Geometry: final body of the model. Coordinates: model frame, mm. A direction names the side the tool comes from. Give positions to 0.01 mm unless a question says otherwise; leave off trailing zeros. Order: outer loops, then holes, each group sorted by start corner. A loop starts at its lowest first (then second) coordinate and runs counter-clockwise, first axis right, second up. Notation, with made-up numbers: (0.25, -24.75) - (56.25, -24.75) arc R28 cw to (56.25, -2.75) - close; hole circle Ø11 at (46.5, 68). An arc over 180 degrees is marked (long way). One line per item, written item: value.
```python
from build123d import *

# Parameters (mm, degrees)
SZKIC1_R                    = 11.5
DODANIE_WYCI_GNI_CIE1_DEPTH = 5


with BuildPart() as part:
    # Szkic1 → Dodanie-wyciągnięcie1 (new body)
    with BuildSketch(Plane.XY):
        with BuildLine():
            Line((61.575587946, -10.709667087), (34.541009179, -0.86988512))
            ThreePointArc((34.541009179, -0.86988512), (16.903048978, 8.361476253), (2.31509692, 21.907963902))
            ThreePointArc((2.31509692, 21.907963902), (0, 23), (-2.31509692, 21.907963902))
            ThreePointArc((-2.31509692, 21.907963902), (-16.903048978, 8.361476253), (-34.541009179, -0.86988512))
            Line((-34.541009179, -0.86988512), (-61.575587946, -10.709667087))
            ThreePointArc((-61.575587946, -10.709667087), (-65.300497868, -16.83130683), (-59.08055809, -20.389645799))
            Line((-59.08055809, -20.389645799), (-32.70655403, -12.827021831))
            ThreePointArc((-32.70655403, -12.827021831), (-21.687864518, -12.201686212), (-11.473608949, -16.381584102))
            ThreePointArc((-11.473608949, -16.381584102), (0, -20), (11.473608949, -16.381584102))
            ThreePointArc((11.473608949, -16.381584102), (21.687864518, -12.201686212), (32.70655403, -12.827021831))
            Line((32.70655403, -12.827021831), (59.08055809, -20.389645799))
            ThreePointArc((59.08055809, -20.389645799), (65.300497868, -16.83130683), (61.575587946, -10.709667087))
        make_face()
        Circle(SZKIC1_R, mode=Mode.SUBTRACT)
    extrude(amount=DODANIE_WYCI_GNI_CIE1_DEPTH)


solid = part.part
```
1) Section B-B, the plane x = 0. Return loops of the section in (y, z).
Answers below:
outline: (-20, 0) - (-11.5, 0) - (-11.5, 5) - (-20, 5) - close; (11.5, 0) - (23, 0) - (23, 5) - (11.5, 5) - close
2) Material intervals for line 1 along Y through (x, z) = (0, 1.7); line 2 along Y through (x, z) = (9.5, 3.85); line 3 along X through (y, z) = (8.5, 4.55), sorted ascending.
Answers below:
line 1: -20 to -11.5, 11.5 to 23
line 2: -17.6 to -6.48, 6.48 to 14.33
line 3: -16.71 to -7.75, 7.75 to 16.71
3) Set-up query: faces 1 (the face through (-46.08, -16.66, 2.46)), 2 (the face through (-16.68, 8.52, 2.46)). Return all of +Z, -Z, +X, -X, +Y, -Y with unobstructed straight access to the full face (end or side cutting, diameter ignored); none if empty.
Answers below:
face 1: +Z, -Z, -Y
face 2: +Z, -Z, -X, +Y
4) First-contact query: pin 1 (2 mm diameter, centred on y = -14.5, z = 1.5, fed in from -X); pin 2 (20.5 mm diameter, centred on x = 0, y = 0, fed in from -Z); pin 3 (3 mm diameter, centred on y = 4.5, z = 3.5, fed in from +X); pin 4 (3 mm diameter, centred on y = 5, z = 4.5, fed in from -X). Flat tips, straight axial feed; report the tip coordinate or a pass-through.
Answers below:
pin 1: x = -65.46
pin 2: through
pin 3: x = 25.72
pin 4: x = -24.77
5) Section C-C, the plane y = 5. Return loops of the section in (x, z).
Answers below:
outline: (-22.1, 0) - (-10.36, 0) - (-10.36, 5) - (-22.1, 5) - close; (10.36, 0) - (22.1, 0) - (22.1, 5) - (10.36, 5) - close
6) Section D-D, the plane x = -17.5. Return loops of the section in (y, z).
Answers below:
outline: (-13.28, 0) - (7.94, 0) - (7.94, 5) - (-13.28, 5) - close
7) Section A-A, the plane z = 2.5. Return loops of the section in (x, y).
Answers below:
outline: (-61.58, -10.71) arc R5 ccw (long way) to (-59.08, -20.39) - (-32.71, -12.83) arc R25 cw to (-11.47, -16.38) arc R20 ccw to (11.47, -16.38) arc R25 cw to (32.71, -12.83) - (59.08, -20.39) arc R5 ccw (long way) to (61.58, -10.71) - (34.54, -0.87) arc R75 cw to (2.32, 21.91) arc R3 ccw to (-2.32, 21.91) arc R75 cw to (-34.54, -0.87) - close; hole circle Ø23 at (0, 0)
8) Mould query, pull axis Y, two halves, no side actions, for faces 3 (the face through (-1.5, 11.4, 2.5)), 4 (the face through (0, 23, 2)), 5 (the face through (45.709, -16.555, 2.465)), 6 (the face through (65.27, -16.94, 2.46)). Classes: released by +Y, released by -Y, zero draft, split by the parting line, or undercut.
Answers below:
face 3: undercut
face 4: released by +Y
face 5: released by -Y
face 6: split by the parting line
